Check sheet for the modelled part. Datum: model origin and axes. Units: mm. Face numbers are marked on the shaded views. A direction names the side the tool comes from. Give positions to 0.01 mm unless a question says otherwise; leave off trailing zeros. Write each loop counter-clockwise with the first axis right and the second up, starting at its lowest first coordinate (ties: lowest second). Pieces come first, ordered by that corner, then holes. Notation, with made-up numbers: (55, 49) -> (107, 49) arc R27 cw to (107, 73) -> close; hole circle Ø7 at (88, -10). An arc over 180 degrees is marked (long way). Answer as a JSON object with one key per item and string values.
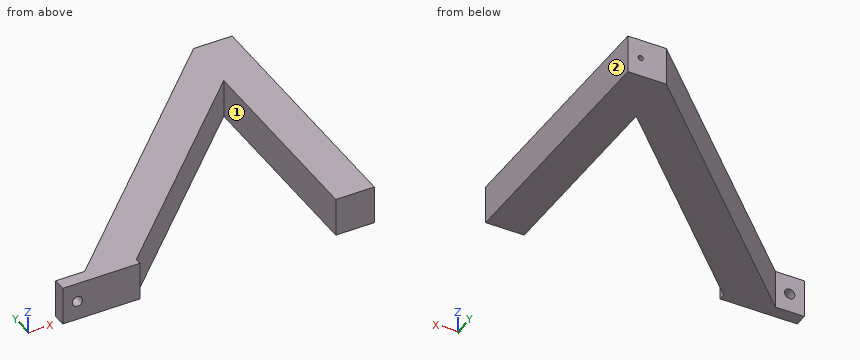
from build123d import *

# Parameters (mm, degrees)
BOSS_EXTRUDE1_DEPTH = 9.525
SKETCH3_R           = 1.27
CUT_EXTRUDE1_DEPTH  = 6.35
SKETCH4_W           = 38.1
SKETCH4_H           = 6.35
BOSS_EXTRUDE2_DEPTH = 19.05
SKETCH5_R           = 2.54
CUT_EXTRUDE3_DEPTH  = 9.525


with BuildPart() as part:
    # Sketch2 → Boss-Extrude1 (new, symmetric)
    with BuildSketch(Plane.XY):
        Polygon((0, 127), (-19.05, 127), (-142.875, 3.175), (-115.934231637, 3.175), (-19.05, 100.059231637), (-19.05, 0), (0, 0), align=None)
    extrude(amount=BOSS_EXTRUDE1_DEPTH, both=True)

    # Sketch3 → Cut-Extrude1 (cut)
    with BuildSketch(Plane(origin=(0, 127, 0), x_dir=(1, 0, 0), z_dir=(0, 1, 0))):
        with Locations(Location((-6.35, 0, 0), (0, 0, 270))):
            Circle(SKETCH3_R)
    extrude(amount=-CUT_EXTRUDE1_DEPTH, mode=Mode.SUBTRACT)

    # Sketch4 → Boss-Extrude2 (add)
    with BuildSketch(Plane.XY.offset(9.525)):
        with Locations((-134.984231637, 3.175)):
            Rectangle(SKETCH4_W, SKETCH4_H)
    extrude(amount=-BOSS_EXTRUDE2_DEPTH)

    # Sketch5 → Cut-Extrude3 (cut)
    with BuildSketch(Plane(origin=(0, 6.35, 0), x_dir=(1, 0, 0), z_dir=(0, 1, 0))):
        with Locations(Location((-146.779052356, 0, 0), (0, 0, 180))):
            Circle(SKETCH5_R)
    extrude(amount=-CUT_EXTRUDE3_DEPTH, mode=Mode.SUBTRACT)


solid = part.part
1. Scan lines: L1, parallel to X at y = 36, z = -1.5; L2, parallel to X at y = 16, z = -7.75; L3, parallel to Y at x = -107, z = 1. Record each from-to range of solid material in increasing order. Write a range as [from, to].
Determined:
{"L1": "[-110.05, -83.11], [-19.05, 0]", "L2": "[-130.05, -103.11], [-19.05, 0]", "L3": "[12.11, 39.05]"}
2. Go/stop test with flat-tipped pins: P1, Ø4, axis at x = -146.78, z = 0, coming from the +Y side; P2, Ø6, axis at y = 47.5, z = -2.5, coming from the -X side; P3, Ø4, axis at x = -94.5, z = 0.5, coming from the +Y side; P4, Ø2, axis at y = 13, z = 1, coming from the -X side. Record where each tip stops, or that it passes through.
Determined:
{"P1": "through", "P2": "x = -101.55", "P3": "y = 53.55", "P4": "x = -134.05"}
3. Sectioned sample at C-C, the plane x = -103. Enter the section's corners in (y, z) (3 decimals).
Determined:
{"outline": "(16.109, -9.525) -> (43.05, -9.525) -> (43.05, 9.525) -> (16.109, 9.525) -> close"}
4. Sectioned sample at A-A, the plane y = 94.5. Enter the section's corners in (x, z) (3 decimals).
Determined:
{"outline": "(-51.55, -9.525) -> (-24.609, -9.525) -> (-24.609, 9.525) -> (-51.55, 9.525) -> close; (-19.05, -9.525) -> (0, -9.525) -> (0, 9.525) -> (-19.05, 9.525) -> close"}
5. Access from +Z, -Z, +X, -X, +Y, -Y to the whole of each face (thin tool, end or side, straight path). Record for the marked faces 1 and 2.
Determined:
{"face 1": "+Z, -Z, -Y", "face 2": "+Z, -Z, +X, +Y, -Y"}
6. Sectioned sample at B-B, the plane z = -5.25. Enter the section's corners in (x, y) (3 decimals).
Determined:
{"outline": "(-154.034, 0) -> (-115.934, 0) -> (-115.934, 3.175) -> (-19.05, 100.059) -> (-19.05, 0) -> (0, 0) -> (0, 127) -> (-19.05, 127) -> (-139.7, 6.35) -> (-154.034, 6.35) -> close"}
